from build123d import *

# Parameters (mm, degrees)
CUT_EXTRUDE1_DEPTH = 20


with BuildPart() as part:
    # Sketch1 → Revolve1 (revolve)
    with BuildSketch(Plane.XY):
        Polygon((0, 0), (0, 9.5), (7, 9.5), (7, 7), (13, 7), (13, 9.5), (20, 9.5), (20, 12.5), (30, 12.5), (30, 10), (130, 10), (130, 0), align=None)
    revolve(axis=Axis((130, 0, 0), (-1, 0, 0)))

    # Sketch2 → Cut-Extrude1 (cut)
    with BuildSketch(Plane(origin=(130, 0, 0), x_dir=(0, 0, -1), z_dir=(1, 0, 0))):
        with BuildLine():
            Line((-9.539392014, 3), (-7.039392014, 3))
            Line((-7.039392014, 3), (-7.039392014, -3))
            Line((-7.039392014, -3), (-9.539392014, -3))
            ThreePointArc((-9.539392014, -3), (-10, 0), (-9.539392014, 3))
        make_face()
    extrude(amount=-CUT_EXTRUDE1_DEPTH, mode=Mode.SUBTRACT)


solid = part.part
For this review, take the finished solid that the model builds, in its own axes (mm). A direction names the side the tool comes from. Round coordinates to 2 decimals unless told otherwise and drop trailing zeros. Order: outer loops, then holes, each group sorted by start corner. A loop starts at its lowest first (then second) coordinate and runs counter-clockwise, first axis right, second up. Notation, with made-up numbers: (62.25, -23.75) -> (92.25, -23.75) arc R29 ccw to (92.25, 5.25) -> close; hole circle Ø11 at (46.5, -6.5). An arc over 180 degrees is marked (long way). Put each result on its own line as item: value.
Q1. Add section A-A on y = 0. Write out the cut boundary in (x, z), plus the area to 3 significant figures.
Check result:
outline: (0, -9.5) -> (7, -9.5) -> (7, -7) -> (13, -7) -> (13, -9.5) -> (20, -9.5) -> (20, -12.5) -> (30, -12.5) -> (30, -10) -> (130, -10) -> (130, 7.04) -> (110, 7.04) -> (110, 10) -> (30, 10) -> (30, 12.5) -> (20, 12.5) -> (20, 9.5) -> (13, 9.5) -> (13, 7) -> (7, 7) -> (7, 9.5) -> (0, 9.5) -> close
area: 2,540 mm2
Q2. Insertion check: pin 1 Ø3 at (y, z) = (9, 8.5) entering from -X; pin 2 Ø8 at (x, z) = (51.5, 0) entering from -Y; pin 3 Ø2 at (x, z) = (85, -9.5) entering from +Y. Each pin has a flat end and moves straight along its axis. Give the tip position at first contact, or say it passes through.
Check result:
pin 1: x = 20
pin 2: y = -10
pin 3: y = 5.27
Q3. Add section B-B on z = 0. Write out the cut boundary in (x, y), plus the area to 3 significant figures.
Check result:
outline: (0, -9.5) -> (7, -9.5) -> (7, -7) -> (13, -7) -> (13, -9.5) -> (20, -9.5) -> (20, -12.5) -> (30, -12.5) -> (30, -10) -> (130, -10) -> (130, 10) -> (30, 10) -> (30, 12.5) -> (20, 12.5) -> (20, 9.5) -> (13, 9.5) -> (13, 7) -> (7, 7) -> (7, 9.5) -> (0, 9.5) -> close
area: 2,600 mm2
Q4. Add section D-D on x = 116.5. Write out the cut boundary in (y, z).
Check result:
outline: (-3, 7.04) -> (-3, 9.54) arc R10 ccw (long way) to (3, 9.54) -> (3, 7.04) -> close
Q5. For probe 1 along X at (y, z) = (6.75, 2.75); probe 2 along X at (y, z) = (-7, 8.75); probe 3 along Y at (x, z) = (29.5, -0.5), list the stretches that pass through material, from the lowest coordinate up. Write a range as [from, to].
Check result:
probe 1: [0, 7], [13, 130]
probe 2: [20, 30]
probe 3: [-12.49, 12.49]
Q6. Mouldability with a two-part tool opening along Y and no side actions: class faces 1 (the cylindrical face through (3.55, 4.38, 8.43)), 2 (the flat face through (0, 0, 0)), 3 (the flat face through (110, 0, 8)) as pulls with the +Y half, pulls with the -Y half, needs draft (parallel to the pull), parting line crosses it, or undercut.
Check result:
face 1: parting line crosses it
face 2: needs draft
face 3: undercut
Q7. Add section C-C on y = 8.25. Write out the cut boundary in (x, z).
Check result:
outline: (0, -4.71) -> (7, -4.71) -> (7, 4.71) -> (0, 4.71) -> close; (13, -4.71) -> (20, -4.71) -> (20, -9.39) -> (30, -9.39) -> (30, -5.65) -> (130, -5.65) -> (130, 5.65) -> (30, 5.65) -> (30, 9.39) -> (20, 9.39) -> (20, 4.71) -> (13, 4.71) -> close
Q8. Machinability: for faces 4 (the cylindrical face through (16.55, 4.38, 8.43)), 5 (the cylindrical face through (80.7, -1.302, -9.915)), 6 (the flat face through (120, 0, 7.039)), which of the approach directions +Z, -Z, +X, -X, +Y, -Y give a long, thin tool a straight path to every point of the face, cutting with its end or side? Answer none if there is none.
Check result:
face 4: -X
face 5: +X
face 6: +Z, +X
